from build123d import *

# Parameters (mm, degrees)
SKETCH2_R                     = 2
BASE_FLANGE1_DEPTH            = 0.7366
EDGE_FLANGE1_STRIP_W          = 4.4196
EDGE_FLANGE1_STRIP_H          = 0.7366
EDGE_FLANGE1_STRIP_CUT_DEPTH  = 15
EDGE_FLANGE1_RELIEF_W         = 4.7879
EDGE_FLANGE1_RELIEF_H         = 0.3683
EDGE_FLANGE1_RELIEF_CUT_DEPTH = 0.7366
EDGE_FLANGE1_DEPTH            = 15
EDGE_FLANGE4_STRIP_W          = 4.4196
EDGE_FLANGE4_STRIP_H          = 0.7366
EDGE_FLANGE4_STRIP_CUT_DEPTH  = 15
EDGE_FLANGE4_RELIEF_W         = 4.7879
EDGE_FLANGE4_RELIEF_H         = 0.3683
EDGE_FLANGE4_RELIEF_CUT_DEPTH = 0.7366
EDGE_FLANGE4_DEPTH            = 15
EDGE_FLANGE5_STRIP_W          = 4.4196
EDGE_FLANGE5_STRIP_H          = 0.7366
EDGE_FLANGE5_STRIP_CUT_DEPTH  = 15
EDGE_FLANGE5_DEPTH            = 15
EDGE_FLANGE6_STRIP_W          = 4.4196
EDGE_FLANGE6_STRIP_H          = 0.7366
EDGE_FLANGE6_STRIP_CUT_DEPTH  = 15
EDGE_FLANGE6_DEPTH            = 15
EDGE_FLANGE7_START            = 56.5
EDGE_FLANGE7_DEPTH            = 15
EDGE_FLANGE7_2_DEPTH          = 15
EDGE_FLANGE8_START            = 56.5
EDGE_FLANGE8_DEPTH            = 15
EDGE_FLANGE8_2_DEPTH          = 15
F_2_0_2_DIAMETER_HOLE4_D      = 2


# Read off the part's stored shape, not the designer's step: Edge-Flange7, Edge-Flange8
# Sheet-metal steps are written as plain solids
with BuildPart() as part:
    # Sketch2 → Base-Flange1 (new body)
    with BuildSketch(Plane.XY):
        with BuildLine():
            Line((-100, 10), (100, 10))
            ThreePointArc((100, 10), (110, 0), (100, -10))
            Line((100, -10), (-100, -10))
            ThreePointArc((-100, -10), (-110, 0), (-100, 10))
        make_face()
        with Locations((100, 0)):
            Circle(SKETCH2_R, mode=Mode.SUBTRACT)
        Circle(SKETCH2_R, mode=Mode.SUBTRACT)
        with Locations((-100, 0)):
            Circle(SKETCH2_R, mode=Mode.SUBTRACT)
    extrude(amount=-BASE_FLANGE1_DEPTH)

    # Edge-Flange1 strip (across the edge) → Edge-Flange1 strip cut (cut)
    with BuildSketch(Plane(origin=(71.5, 10, 0), x_dir=(0, -1, 0), z_dir=(-1, 0, 0))):
        with Locations((-1.4732, -0.3683)):
            Rectangle(EDGE_FLANGE1_STRIP_W, EDGE_FLANGE1_STRIP_H)
    extrude(amount=EDGE_FLANGE1_STRIP_CUT_DEPTH, mode=Mode.SUBTRACT)

    # Edge-Flange1 relief (on the sheet) → Edge-Flange1 relief cut (cut)
    with BuildSketch(Plane(origin=(71.5, 9.2634, 0), x_dir=(0, -1, 0), z_dir=(0, 0, 1))):
        with Locations((-2.02565, 0.18415)):
            Rectangle(EDGE_FLANGE1_RELIEF_W, EDGE_FLANGE1_RELIEF_H)
        with Locations((-2.02565, -15.18415)):
            Rectangle(EDGE_FLANGE1_RELIEF_W, EDGE_FLANGE1_RELIEF_H)
    extrude(amount=-EDGE_FLANGE1_RELIEF_CUT_DEPTH, mode=Mode.SUBTRACT)

    # Edge-Flange1 section (across the edge) → Edge-Flange1 (add)
    with BuildSketch(Plane(origin=(71.5, 10, 0), x_dir=(0, -1, 0), z_dir=(-1, 0, 0))):
        with BuildLine():
            Line((-0.7366, 0.7366), (-0.7366, 15))
            Line((-0.7366, 15), (0, 15))
            Line((0, 15), (0, 0.7366))
            ThreePointArc((0, 0.7366), (0.215745145, 0.215745145), (0.7366, 0))
            Line((0.7366, 0), (0.7366, -0.7366))
            ThreePointArc((0.7366, -0.7366), (-0.30510971, -0.30510971), (-0.7366, 0.7366))
        make_face()
    extrude(amount=EDGE_FLANGE1_DEPTH)

    # Edge-Flange4 strip (across the edge) → Edge-Flange4 strip cut (cut)
    with BuildSketch(Plane(origin=(56.5, -10, 0), x_dir=(0, 1, 0), z_dir=(1, 0, 0))):
        with Locations((-1.4732, -0.3683)):
            Rectangle(EDGE_FLANGE4_STRIP_W, EDGE_FLANGE4_STRIP_H)
    extrude(amount=EDGE_FLANGE4_STRIP_CUT_DEPTH, mode=Mode.SUBTRACT)

    # Edge-Flange4 relief (on the sheet) → Edge-Flange4 relief cut (cut)
    with BuildSketch(Plane(origin=(56.5, -9.2634, 0), x_dir=(0, 1, 0), z_dir=(0, 0, 1))):
        with Locations((-2.02565, 0.18415)):
            Rectangle(EDGE_FLANGE4_RELIEF_W, EDGE_FLANGE4_RELIEF_H)
        with Locations((-2.02565, -15.18415)):
            Rectangle(EDGE_FLANGE4_RELIEF_W, EDGE_FLANGE4_RELIEF_H)
    extrude(amount=-EDGE_FLANGE4_RELIEF_CUT_DEPTH, mode=Mode.SUBTRACT)

    # Edge-Flange4 section (across the edge) → Edge-Flange4 (add)
    with BuildSketch(Plane(origin=(56.5, -10, 0), x_dir=(0, 1, 0), z_dir=(1, 0, 0))):
        with BuildLine():
            Line((-0.7366, 0.7366), (-0.7366, 15))
            Line((-0.7366, 15), (0, 15))
            Line((0, 15), (0, 0.7366))
            ThreePointArc((0, 0.7366), (0.215745145, 0.215745145), (0.7366, 0))
            Line((0.7366, 0), (0.7366, -0.7366))
            ThreePointArc((0.7366, -0.7366), (-0.30510971, -0.30510971), (-0.7366, 0.7366))
        make_face()
    extrude(amount=EDGE_FLANGE4_DEPTH)

    # Edge-Flange5 strip (across the edge) → Edge-Flange5 strip cut (cut)
    with BuildSketch(Plane(origin=(71.5, 10, 15), x_dir=(0, 0, -1), z_dir=(-1, 0, 0))):
        with Locations((-1.4732, -0.3683)):
            Rectangle(EDGE_FLANGE5_STRIP_W, EDGE_FLANGE5_STRIP_H)
    extrude(amount=EDGE_FLANGE5_STRIP_CUT_DEPTH, mode=Mode.SUBTRACT)

    # Edge-Flange5 section (across the edge) → Edge-Flange5 (add)
    with BuildSketch(Plane(origin=(71.5, 10, 15), x_dir=(0, 0, -1), z_dir=(-1, 0, 0))):
        with BuildLine():
            Line((-0.7366, 0.7366), (-0.7366, 9.99))
            Line((-0.7366, 9.99), (0, 9.99))
            Line((0, 9.99), (0, 0.7366))
            ThreePointArc((0, 0.7366), (0.215745145, 0.215745145), (0.7366, 0))
            Line((0.7366, 0), (0.7366, -0.7366))
            ThreePointArc((0.7366, -0.7366), (-0.30510971, -0.30510971), (-0.7366, 0.7366))
        make_face()
    extrude(amount=EDGE_FLANGE5_DEPTH)

    # Edge-Flange6 strip (across the edge) → Edge-Flange6 strip cut (cut)
    with BuildSketch(Plane(origin=(56.5, -10, 15), x_dir=(0, 0, -1), z_dir=(1, 0, 0))):
        with Locations((-1.4732, -0.3683)):
            Rectangle(EDGE_FLANGE6_STRIP_W, EDGE_FLANGE6_STRIP_H)
    extrude(amount=EDGE_FLANGE6_STRIP_CUT_DEPTH, mode=Mode.SUBTRACT)

    # Edge-Flange6 section (across the edge) → Edge-Flange6 (add)
    with BuildSketch(Plane(origin=(56.5, -10, 15), x_dir=(0, 0, -1), z_dir=(1, 0, 0))):
        with BuildLine():
            Line((-0.7366, 0.7366), (-0.7366, 10))
            Line((-0.7366, 10), (0, 10))
            Line((0, 10), (0, 0.7366))
            ThreePointArc((0, 0.7366), (0.215745145, 0.215745145), (0.7366, 0))
            Line((0.7366, 0), (0.7366, -0.7366))
            ThreePointArc((0.7366, -0.7366), (-0.30510971, -0.30510971), (-0.7366, 0.7366))
        make_face()
    extrude(amount=EDGE_FLANGE6_DEPTH)

    # Edge-Flange7 outline → Edge-Flange7 (cut)
    with BuildSketch(Plane.YZ.offset(EDGE_FLANGE7_START)):
        with BuildLine():
            Line((0, 15.7366), (-0.197371375, 15.7366))
            ThreePointArc((-0.197371375, 15.7366), (-0.7366, 15.197371375), (-1.4732, 15))
            Line((-1.4732, 15), (0, 15))
            Line((0, 15), (0, 15.7366))
        make_face()
    extrude(amount=EDGE_FLANGE7_DEPTH, mode=Mode.SUBTRACT)

    # Edge-Flange7 2 outline → Edge-Flange7 2 (add)
    with BuildSketch(Plane.YZ.offset(EDGE_FLANGE7_START)):
        with BuildLine():
            ThreePointArc((-0.197371375, 15.7366), (-0.050198073, 16.091907783), (0, 16.4732))
            Line((0, 16.4732), (0, 20.7366))
            Line((0, 20.7366), (-0.7366, 20.7366))
            Line((-0.7366, 20.7366), (-0.7366, 16.4732))
            ThreePointArc((-0.7366, 16.4732), (-0.952345145, 15.952345145), (-1.4732, 15.7366))
            Line((-1.4732, 15.7366), (-0.197371375, 15.7366))
        make_face()
    extrude(amount=EDGE_FLANGE7_2_DEPTH)

    # Edge-Flange8 outline → Edge-Flange8 (cut)
    with BuildSketch(Plane.YZ.offset(EDGE_FLANGE8_START)):
        with BuildLine():
            ThreePointArc((1.4832, 15), (0.7466, 15.197371375), (0.207371375, 15.7366))
            Line((0.207371375, 15.7366), (0.01, 15.7366))
            Line((0.01, 15.7366), (0.01, 15))
            Line((0.01, 15), (1.4832, 15))
        make_face()
    extrude(amount=EDGE_FLANGE8_DEPTH, mode=Mode.SUBTRACT)

    # Edge-Flange8 2 outline → Edge-Flange8 2 (add)
    with BuildSketch(Plane.YZ.offset(EDGE_FLANGE8_START)):
        with BuildLine():
            Line((0.7466, 20.7366), (0.01, 20.7366))
            Line((0.01, 20.7366), (0.01, 16.4732))
            ThreePointArc((0.01, 16.4732), (0.060198073, 16.091907783), (0.207371375, 15.7366))
            Line((0.207371375, 15.7366), (1.4832, 15.7366))
            ThreePointArc((1.4832, 15.7366), (0.962345145, 15.952345145), (0.7466, 16.4732))
            Line((0.7466, 16.4732), (0.7466, 20.7366))
        make_face()
    extrude(amount=EDGE_FLANGE8_2_DEPTH)

    # Ø2.0 (2) Diameter Hole4 (through all)
    with Locations(Plane(origin=(0, 0.7466, 0), x_dir=(1, 0, 0), z_dir=(0, 1, 0))):
        with Locations((61.5, -18.907246823)):
            Hole(F_2_0_2_DIAMETER_HOLE4_D / 2)


solid = part.part
For this review, take the finished solid that the model builds, in its own axes (mm). A direction names the side the tool comes from. Coordinates: 2 decimals unless noted, no trailing zeros. Order: outer loops, then holes, each group sorted by start corner. A loop starts at its lowest first (then second) coordinate and runs counter-clockwise, first axis right, second up. Notation, with made-up numbers: (1.5, 42) - (23.5, 42) arc R6 ccw to (23.5, 49) - close; hole circle Ø11 at (39.5, 87). An arc over 180 degrees is marked (long way). Use one line per item in the form item = value.
Q1. Consider section C-C (x = 69.5). Give the boundary of the cut face in (y, z).
Checked values:
outline = (-10.74, 0.74) arc R1.47 ccw to (-9.26, -0.74) - (9.26, -0.74) arc R1.47 ccw to (10.74, 0.74) - (10.74, 14.26) arc R1.47 ccw to (9.26, 15.74) - (1.48, 15.74) arc R0.74 cw to (0.75, 16.47) - (0.75, 20.74) - (0.01, 20.74) - (0.01, 16.47) arc R1.47 ccw to (1.48, 15) - (9.26, 15) arc R0.74 cw to (10, 14.26) - (10, 0.74) arc R0.74 cw to (9.26, 0) - (-9.26, 0) arc R0.74 cw to (-10, 0.74) - (-10, 14.26) arc R0.74 cw to (-9.26, 15) - (-1.47, 15) arc R1.47 ccw to (0, 16.47) - (0, 20.74) - (-0.74, 20.74) - (-0.74, 16.47) arc R0.74 cw to (-1.47, 15.74) - (-9.26, 15.74) arc R1.47 ccw to (-10.74, 14.26) - close
Q2. Consider section A-A (x = 0). Give the boundary of the cut face in (y, z).
Checked values:
outline = (-10, -0.74) - (-2, -0.74) - (-2, 0) - (-10, 0) - close; (2, -0.74) - (10, -0.74) - (10, 0) - (2, 0) - close
Q3. For P1, Ø1.3, axis at x = 67, z = 19.5, coming from the -Y side; P2, Ø1, axis at x = -6, y = 3, coming from the +Z side; P3, Ø0.6, axis at y = 9.5, z = -0.5, coming from the +X side; P4, Ø5.5, axis at y = -5.5, z = 5.5, coming from the +X side, all flat-tipped, find the tip position at first contact; note any pin that passes through.
Checked values:
P1 = -0.74
P2 = 0
P3 = 103.92
P4 = through
Q4. For probe 1 along Y at (x, z) = (-100, -0.5); probe 2 along Z at (x, y) = (-77.5, -8); probe 3 along Z at (x, y) = (61.5, -0.3), list the stretches that pass through material, from the lowest coordinate up. Write a range as from..to.
Checked values:
probe_1 = -10..-2, 2..10
probe_2 = -0.74..0
probe_3 = -0.74..0, 15.58..17.91, 19.91..20.74
Q5. Draft analysis for pull direction Y (two halves, no side actions). For faces 1 (the flat face through (64, -5, 15.737)), 2 (the flat face through (64, 5, 15)), 3 (the flat face through (64, 0.747, 19)), state which applies: +Y half, -Y half, draft (parallel to the pull), parting line (faces both ways), or undercut.
Checked values:
face_1 = draft
face_2 = undercut
face_3 = +Y half
Q6. For faces 4 (the flat face through (64, 5, 15.737)), 5 (the flat face through (64, -10, 8)), 6 (the flat face through (64, -10.737, 7)), list the 3-axis set-ups (+Z, -Z, +X, -X, +Y, -Y) from which the entire face can be reached by the end or side of a thin tool; tool diameter is ignored.
Checked values:
face_4 = +Z, +X, -X, +Y
face_5 = +X, -X
face_6 = +Z, -Z, +X, -X, -Y
Q7. Consider section B-B (z = 10). Give the boundary of the cut face in (x, y), then the cut area to 3 significant figures.
Checked values:
outline = (56.5, -10.74) - (71.5, -10.74) - (71.5, -10) - (56.5, -10) - close; (56.5, 10) - (71.5, 10) - (71.5, 10.74) - (56.5, 10.74) - close
area = 22.1 mm2
